Input: part model. Units: mm. Frame: model coordinates. A direction names the side the tool comes from. Coordinates: 2 decimals unless noted, no trailing zeros. Write each loop counter-clockwise with the first axis right and the second up, starting at its lowest first coordinate (ties: lowest second). Pieces come first, ordered by that corner, then holes.
1) Section query A-A (z = 2.95). Output: boundary loops of the cut face in (x, y), then the cut area to 4 significant figures.
2) Section query C-C (y = 50). Output: boundary loops of the cut face in (x, z), then the cut area to 3 significant figures.
3) Pin query (flat end, axial travel): pin 1 Ø1.8 at (x, z) = (101.5, 2) entering from -Y; pin 2 Ø1 at (y, z) = (11, 1) entering from -X; pin 3 Ø1 at (x, z) = (138.5, 2.5) entering from -Y. Return the tip coordinate at first contact, or that it passes through.
4) Set-up query: faces 1 (the flat face through (138, 45, 2)), 2 (the flat face through (0, 7, 2)), 3 (the flat face through (136, 7, 2)), 4 (the flat face through (0, 52, 2)), 5 (the flat face through (67, 60, 2)). Return all of +Z, -Z, +X, -X, +Y, -Y with unobstructed straight access to the full face (end or side cutting, diameter ignored); none if empty.
5) Line query: L1, parallel to Y at x = 3.5, z = 2.55; L2, parallel to X at y = 2.5, z = 2.9. Output: solid intervals per line, ascending.
6) Section query B-B (x = 108). Output: boundary loops of the cut face in (y, z).
from build123d import *

# Parameters (mm, degrees)
SKETCH_1_W      = 136
SKETCH_1_H      = 60
SKETCH_1_W_2    = 3.5
SKETCH_1_H_2    = 30
SKETCH_1_W_3    = 30
SKETCH_1_H_3    = 3.5
EXTRUDE_1_DEPTH = 3.5


with BuildPart() as part:
    # Эскиз1 → Бобышка-Вытянуть1 (new body)
    with BuildSketch(Plane.XY):
        with Locations((68, 30)):
            Rectangle(SKETCH_1_W, SKETCH_1_H)
        with Locations((-1.75, 30)):
            Rectangle(SKETCH_1_W_2, SKETCH_1_H_2)
        with Locations((137.75, 30)):
            Rectangle(SKETCH_1_W_2, SKETCH_1_H_2)
        with Locations((68, -1.75)):
            Rectangle(SKETCH_1_W_3, SKETCH_1_H_3)
    extrude(amount=EXTRUDE_1_DEPTH)


solid = part.part
Answer:
1. outline: (-3.5, 15) - (0, 15) - (0, 0) - (53, 0) - (53, -3.5) - (83, -3.5) - (83, 0) - (136, 0) - (136, 15) - (139.5, 15) - (139.5, 45) - (136, 45) - (136, 60) - (0, 60) - (0, 45) - (-3.5, 45) - close
1. area: 8,475 mm2
2. outline: (0, 0) - (136, 0) - (136, 3.5) - (0, 3.5) - close
2. area: 476 mm2
3. pin 1: stops at y = 0
3. pin 2: stops at x = 0
3. pin 3: stops at y = 15
4. face 1: +Z, -Z, +X, +Y
4. face 2: +Z, -Z, -X, -Y
4. face 3: +Z, -Z, +X, -Y
4. face 4: +Z, -Z, -X, +Y
4. face 5: +Z, -Z, +X, -X, +Y
5. L1: y = 0 to 60
5. L2: x = 0 to 136
6. outline: (0, 0) - (60, 0) - (60, 3.5) - (0, 3.5) - close
